```python
from build123d import *

# Parameters (mm, degrees)
ESBO_O1_R                = 4
RESSALTO_EXTRUS_O1_DEPTH = 4
ESBO_O3_R                = 4
RESSALTO_EXTRUS_O2_DEPTH = 2.5
ESBO_O5_R                = 2.5
CORTE_EXTRUS_O1_DEPTH    = 5.5


with BuildPart() as part:
    # Esboço1 → Ressalto-extrusão1 (new body)
    with BuildSketch(Plane.XY):
        with Locations((25, 0.5)):
            Circle(ESBO_O1_R)
        with BuildLine():
            ThreePointArc((0.394172842, -0.77044566), (1.648131789, 0.085177798), (3.16042427, 0.217374592))
            Line((3.16042427, 0.217374592), (23.676638803, -3.27474703))
            ThreePointArc((23.676638803, -3.27474703), (21.056715321, 1.171197392), (25, 4.5))
            Line((25, 4.5), (7.714247019, 9.781757855))
            ThreePointArc((7.714247019, 9.781757855), (6.991805383, 9.945138485), (6.253154341, 10))
            Line((6.253154341, 10), (1.5, 10))
            ThreePointArc((1.5, 10), (-5.217514421, 7.217514421), (-8, 0.5))
            Line((-8, 0.5), (-8, -0.5))
            ThreePointArc((-8, -0.5), (-7.713418989, -2.815795873), (-6.870966205, -4.991873194))
            ThreePointArc((-6.870966205, -4.991873194), (-5.331925608, -6.033714451), (-3.600088608, -5.359311184))
            Line((-3.600088608, -5.359311184), (0.394172842, -0.77044566))
        make_face()
    extrude(amount=RESSALTO_EXTRUS_O1_DEPTH)

    # Esboço3 → Ressalto-extrusão2 (add)
    with BuildSketch(Plane.XY.offset(4)):
        with Locations(Location((25, 0.5, 0), (0, 0, 250.680213843))):
            Circle(ESBO_O3_R)
    extrude(amount=RESSALTO_EXTRUS_O2_DEPTH)

    # Esboço5 → Corte-extrusão1 (cut)
    with BuildSketch(Plane.XY.offset(6.5)):
        with Locations((25, 0.5)):
            Circle(ESBO_O5_R)
    extrude(amount=-CORTE_EXTRUS_O1_DEPTH, mode=Mode.SUBTRACT)


solid = part.part
```
Geometry check sheet. Reference: the model listing, model coordinates, mm. A direction names the side the tool comes from. Coordinates: 2 decimals unless noted, no trailing zeros. Order: outer loops, then holes, each group sorted by start corner. A loop starts at its lowest first (then second) coordinate and runs counter-clockwise, first axis right, second up. Notation, with made-up numbers: M 20.25,-24 L 72.25,-24 A17 ccw 72.25,-2 Z; hole C 86,-20 d5. An arc over 180 degrees is marked long. Answer as a JSON object with one key per item and string values.
Q1. Cross-section at A-A on z = 2. Record the cut outline in (x, y), and give its area (3 significant figures).
Results are:
{"outline": "M -8,-0.5 A9.5 ccw -6.87,-4.99 A2 ccw -3.6,-5.36 L 0.39,-0.77 A3 cw 3.16,0.22 L 23.68,-3.27 A4 ccw long 25,4.5 L 7.71,9.78 A5 ccw 6.25,10 L 1.5,10 A9.5 ccw -8,0.5 Z; hole C 25,0.5 d5", "area": "338 mm²"}
Q2. Depth check by flat-ended pin: pin 1 Ø2 at (x, z) = (10, 2) entering from -Y. Enter the tip coordinate at first touch or a pass-through.
Results are:
{"pin 1": "stops at y = -1.12"}
Q3. Cross-section at D-D on z = 5.5. Record the cut outline in (x, y).
Results are:
{"outline": "C 25,0.5 d8; hole C 25,0.5 d5"}
Q4. Tool access check on faces 5 (the flat face through (13.275, -1.504, 1.972)), 6 (the cylindrical face through (23, 2, 4)), 7 (the cylindrical face through (-7.721, -2.784, 1.972)). Record the directions out of +Z, -Z, +X, -X, +Y, -Y that give a thin tool (end or side, any length) a straight path to the whole face; none if there is none.
Results are:
{"face 5": "+Z, -Z, -Y", "face 6": "+Z", "face 7": "+Z, -Z, -X, -Y"}
Q5. Release check for a two-part mould opening along Y. For faces 1 (the flat face through (25, 1, 1)), 2 (the flat face through (16.478, 7.104, 1.972)), 3 (the flat face through (5, 4, 4)), 4 (the cylindrical face through (-5.36, -6.03, 1.97)) record: released by +Y, released by -Y, zero draft, split by the parting line, or undercut.
Results are:
{"face 1": "undercut", "face 2": "released by +Y", "face 3": "zero draft", "face 4": "released by -Y"}
Q6. Cross-section at C-C on x = 11. Record the cut outline in (y, z), and give its area (3 significant figures).
Results are:
{"outline": "M -1.12,0 L 8.78,0 L 8.78,4 L -1.12,4 Z", "area": "39.6 mm²"}
Q7. Scan lines: line 1 (Y direction, x = 25, z = 2.6); line 2 (Z direction, x = 25, y = -0.75); line 3 (Y direction, x = 27, z = 2.5). Record each from-to range of solid material in increasing order.
Results are:
{"line 1": "y = -3.5 to -2, 3 to 4.5", "line 2": "z = 0 to 1", "line 3": "y = -2.96 to -1, 2 to 3.96"}
Q8. Cross-section at B-B on y = 8.75. Record the cut outline in (x, z).
Results are:
{"outline": "M -3.21,0 L 11.09,0 L 11.09,4 L -3.21,4 Z"}
